Can you work these out from the model? Positions are in its coordinate system, mm. Coordinates: 2 decimals unless noted, no trailing zeros. Order: outer loops, then holes, each group sorted by start corner. A loop starts at its lowest first (then second) coordinate and runs counter-clockwise, first axis right, second up. Notation, with made-up numbers: (57.25, 74.5) -> (70.25, 74.5) arc R18 ccw to (70.25, 87.5) -> close; hole circle Ø4 at (36.5, 7.5). An arc over 180 degrees is marked (long way). Answer as CSV lines item,"result".
from build123d import *

# Parameters (mm, degrees)
ESQUISSE1_R             = 3
BOSS_EXTRU_1_DEPTH      = 200
ESQUISSE4_W             = 5
ESQUISSE4_H             = 50
BOSS_EXTRU_4_DEPTH      = 180
BOSS_EXTRU_7_DEPTH      = 50
ESQUISSE6_W             = 20
ESQUISSE6_H             = 10.719834163
ENL_V_MAT_EXTRU_2_DEPTH = 10
ESQUISSE5_W             = 10
ESQUISSE5_H             = 10
ENL_V_MAT_EXTRU_1_DEPTH = 10
ESQUISSE14_R            = 5
ENL_V_MAT_EXTRU_4_DEPTH = 15
BOSS_EXTRU_8_REACH      = 242.401
ENL_V_MAT_EXTRU_5_REACH = 238.046
ESQUISSE16_W            = 190
ESQUISSE16_H            = 60


with BuildPart() as part:
    # Esquisse1 → Boss.-Extru.1 (new body)
    with BuildSketch(Plane.XY):
        Polygon((-105.796013405, 0), (84.203986595, 0), (84.203986595, 33.502126335), (-105.796013405, 2), align=None)
        with Locations((69.406004871, 22.939397164)):
            Circle(ESQUISSE1_R, mode=Mode.SUBTRACT)
        with Locations((40.981469067, 6.77616521)):
            Circle(ESQUISSE1_R, mode=Mode.SUBTRACT)
        with Locations((-40.796013405, 6)):
            Circle(ESQUISSE1_R, mode=Mode.SUBTRACT)
        with Locations((8.861542866, 12.901085106)):
            Circle(ESQUISSE1_R, mode=Mode.SUBTRACT)
    extrude(amount=BOSS_EXTRU_1_DEPTH)

    # Esquisse4 → Boss.-Extru.4 (add)
    with BuildSketch(Plane(origin=(84.203986595, 0, 0), x_dir=(0, 0, -1), z_dir=(1, 0, 0))):
        with Locations((-202.5, 25)):
            Rectangle(ESQUISSE4_W, ESQUISSE4_H)
        with Locations((2.5, 25)):
            Rectangle(ESQUISSE4_W, ESQUISSE4_H)
    extrude(amount=-BOSS_EXTRU_4_DEPTH)

    # Esquisse8 → Boss.-Extru.7 (add)
    with BuildSketch(Plane(origin=(0, 50, 0), x_dir=(1, 0, 0), z_dir=(0, 1, 0))):
        Polygon((84.203986595, 0), (-95.796013405, 0), (-95.796013405, -5), align=None)
    boss_extru_7 = extrude(amount=-BOSS_EXTRU_7_DEPTH)

    # Esquisse6 → Enlèv. mat.-Extru.2 (cut)
    with BuildSketch(Plane(origin=(0, 0, -5), x_dir=(-1, 0, 0), z_dir=(0, 0, -1))):
        with Locations((95.796013405, 5.359917081)):
            Rectangle(ESQUISSE6_W, ESQUISSE6_H)
    enl_v_mat_extru_2 = extrude(amount=-ENL_V_MAT_EXTRU_2_DEPTH, mode=Mode.SUBTRACT)

    # Esquisse5 → Enlèv. mat.-Extru.1 (cut)
    with BuildSketch(Plane(origin=(84.203986595, 0, 0), x_dir=(0, 0, -1), z_dir=(1, 0, 0))):
        with Locations((-200, 5)):
            Rectangle(ESQUISSE5_W, ESQUISSE5_H)
        with Locations((0, 5)):
            Rectangle(ESQUISSE5_W, ESQUISSE5_H)
    extrude(amount=-ENL_V_MAT_EXTRU_1_DEPTH, mode=Mode.SUBTRACT)

    # Esquisse14 → Enlèv. mat.-Extru.4 (cut)
    with BuildSketch(Plane(origin=(0, 0, -5), x_dir=(-1, 0, 0), z_dir=(0, 0, -1))):
        with Locations((-69.406004871, 22.939397164)):
            Circle(ESQUISSE14_R)
        with Locations((-40.981469067, 6.77616521)):
            Circle(ESQUISSE14_R)
        with Locations((-8.861542866, 12.901085106)):
            Circle(ESQUISSE14_R)
        with Locations((40.796013405, 6)):
            Circle(ESQUISSE14_R)
    enl_v_mat_extru_4 = extrude(amount=-ENL_V_MAT_EXTRU_4_DEPTH, mode=Mode.SUBTRACT)

    # Symétrie3: Boss.-Extru.7, Enlèv. mat.-Extru.2, Enlèv. mat.-Extru.4 across plane
    add(boss_extru_7.mirror(Plane(origin=(0, 0, 100), x_dir=(1, 0, 0), z_dir=(0, 0, -1))))
    add(enl_v_mat_extru_2.mirror(Plane(origin=(0, 0, 100), x_dir=(1, 0, 0), z_dir=(0, 0, -1))), mode=Mode.SUBTRACT)
    add(enl_v_mat_extru_4.mirror(Plane(origin=(0, 0, 100), x_dir=(1, 0, 0), z_dir=(0, 0, -1))), mode=Mode.SUBTRACT)

    # Boss.-Extru.8: up to this plane
    boss_extru_8_end = Plane(origin=(-95.796013405, -180.069431054, 195), z_dir=(-0.0277670672403533, 0, 0.9996144206527183))
    # Esquisse15 → Boss.-Extru.8 (add, up to the surface)
    with BuildSketch(Plane(origin=(0, 0, -5), x_dir=(-1, 0, 0), z_dir=(0, 0, -1)), mode=Mode.PRIVATE) as boss_extru_8_sk1:
        Polygon((-84.203986595, 33.502126335), (-79.203986595, 32.67312301), (-79.203986595, 50), (-84.203986595, 50), align=None)
    boss_extru_8_tool1 = split(extrude(boss_extru_8_sk1.sketch, amount=-BOSS_EXTRU_8_REACH, mode=Mode.PRIVATE), bisect_by=boss_extru_8_end, keep=Keep.BOTH, mode=Mode.PRIVATE)
    add(boss_extru_8_tool1.solids().sort_by_distance((81.683563, 41.542119, -5))[0])

    # Enlèv. mat.-Extru.5: up to this face of the body (flat: up to its plane)
    enl_v_mat_extru_5_end = Plane(part.part.faces().sort_by_distance((-10.38578146, 0, 100.003530671))[0])
    # Esquisse16 → Enlèv. mat.-Extru.5 (cut, up to the picked face)
    with BuildSketch(Plane(origin=(0, 50, 0), x_dir=(1, 0, 0), z_dir=(0, 1, 0)), mode=Mode.PRIVATE) as enl_v_mat_extru_5_sk1:
        with Locations((-10.796013405, -175)):
            Rectangle(ESQUISSE16_W, ESQUISSE16_H)
    enl_v_mat_extru_5_tool1 = split(extrude(enl_v_mat_extru_5_sk1.sketch, amount=-ENL_V_MAT_EXTRU_5_REACH, mode=Mode.PRIVATE), bisect_by=enl_v_mat_extru_5_end, keep=Keep.BOTH, mode=Mode.PRIVATE)
    # Esquisse16 → Enlèv. mat.-Extru.5 (cut, up to the picked face)
    with BuildSketch(Plane(origin=(0, 50, 0), x_dir=(1, 0, 0), z_dir=(0, 1, 0)), mode=Mode.PRIVATE) as enl_v_mat_extru_5_sk2:
        with Locations((-10.796013405, -25)):
            Rectangle(ESQUISSE16_W, ESQUISSE16_H)
    enl_v_mat_extru_5_tool2 = split(extrude(enl_v_mat_extru_5_sk2.sketch, amount=-ENL_V_MAT_EXTRU_5_REACH, mode=Mode.PRIVATE), bisect_by=enl_v_mat_extru_5_end, keep=Keep.BOTH, mode=Mode.PRIVATE)
    add(enl_v_mat_extru_5_tool1.solids().sort_by(Axis((-10.796013, 50, 175), (0, -1, 0)))[0], mode=Mode.SUBTRACT)
    add(enl_v_mat_extru_5_tool2.solids().sort_by(Axis((-10.796013, 50, 25), (0, -1, 0)))[0], mode=Mode.SUBTRACT)


solid = part.part
Q1. Imagine slicing it at B-B (x = 62.5). List the corners of the cut face in (y, z) for me, and give its area (3 significant figures).
Solution:
outline,"(0, 55) -> (29.9, 55) -> (29.9, 145) -> (0, 145) -> close"
area,"2,690 mm2"
Q2. If I drill on line 1 (X direction, y = 41.5, z = 88.5); line 2 (Y direction, x = 40, z = 115.5); line 3 (Y direction, x = -58, z = 141.5), over which ranges is the centre line in solid material (lowest first)?
Solution:
line 1,"79.2 to 84.2"
line 2,"0 to 3.94, 9.61 to 26.17"
line 3,"0 to 9.92"
Q3. For P1, Ø5, axis at y = 44.5, z = 111.5, coming from the -X side; P2, Ø1.5, axis at x = -21, z = 95.5, coming from the +Y side, each with a flat end and sliding along its axis, tell me the tip position at first contact or that it passes through.
Solution:
P1,"x = 79.2"
P2,"y = 16.18"
Q4. Imagine slicing it at A-A (z = 105). List the corners of the cut face in (x, y) for me, and give its area (3 significant figures).
Solution:
outline,"(-105.8, 0) -> (84.2, 0) -> (84.2, 50) -> (79.2, 50) -> (79.2, 32.67) -> (-105.8, 2) -> close; hole circle Ø6 at (-40.8, 6); hole circle Ø6 at (8.86, 12.9); hole circle Ø6 at (40.98, 6.78); hole circle Ø6 at (69.41, 22.94)"
area,"3,340 mm2"
Q5. Imagine slicing it at C-C (x = -21). List the corners of the cut face in (y, z) for me.
Solution:
outline,"(0, 55) -> (16.06, 55) -> (16.06, 145) -> (0, 145) -> close"
Q6. We'd pull the mould along X, two halves only. Please class faces 1 (the cylindrical face through (66.41, 23.07, 99.37)), 2 (the flat face through (79.204, 41, 99)), 3 (the flat face through (-9, 0, 101)), 4 (the flat face through (84.204, 25, 101)): pulls with the +X half, pulls with the -X half, needs draft (parallel to the pull), parting line crosses it, or undercut.
Solution:
face 1,"undercut"
face 2,"pulls with the -X half"
face 3,"needs draft"
face 4,"pulls with the +X half"
